Autodesk Inventor part; units mm, degrees
ref_plane "YZ Plane" through (0, 0, 0) normal (1, 0, 0) x (0, 1, 0)
ref_plane "XZ Plane" through (0, 0, 0) normal (0, 1, 0) x (-1, 0, 0)
ref_plane "XY Plane" through (0, 0, 0) normal (0, 0, 1) x (1, 0, 0)
sketch "Sketch1" plane through (0, 0, 0) normal (0, 1, 0) x (-1, 0, 0)
  line L0 (0, 0) -> (0, 20.8)
  line L1 (0, 20.8) -> (-2, 20.8)
  line L2 (-2, 20.8) -> (-2, 14.8)
  line L3 (-2, 14.8) -> (-3, 14.8)
  line L4 (-3, 14.8) -> (-3, 2.8)
  line L5 (-3, 2.8) -> (-5, 2.8)
  line L6 (-5, 2.8) -> (-5, 0)
  line L7 (-5, 0) -> (0, 0)
  dimension "d0" = 10
  dimension "d1" = 6
  dimension "d2" = 4
  dimension "d3" = 6
  dimension "d4" = 12
  dimension "d5" = 2.8
revolve "Revolution1" add sketch "Sketch1" angle 360 about axis through (0, 0, 0) along (0, 0, 1)
thread "Thread1"
sketch "Sketch2" plane through (0, 0, 0) normal (0, 0, -1) x (-1, 0, 0)
  line L0 (0, 1.4434) -> (1.25, 0.7217)
  line L1 (1.25, 0.7217) -> (1.25, -0.7217)
  line L2 (1.25, -0.7217) -> (0, -1.4434)
  line L3 (0, -1.4434) -> (-1.25, -0.7217)
  line L4 (-1.25, -0.7217) -> (-1.25, 0.7217)
  line L5 (-1.25, 0.7217) -> (0, 1.4434)
  point P0 (0, 0)
  point P1 (0, 0)
  dimension "d9" = 2.5
extrude "Extrusion1" cut sketch "Sketch2" against normal blind 2
chamfer "Chamfer1" distance 0.43 angle 45 1 edges at (-2, 0, 20.8)
properties part number "DBTSY4-12-6-DHC" material "Stainless Steel AISI 304"
Model file for the job. Use its own axes, mm. A direction names the side the tool comes from. Give positions to 0.01 mm unless a question says otherwise; leave off trailing zeros. Order: outer loops, then holes, each group sorted by start corner. A loop starts at its lowest first (then second) coordinate and runs counter-clockwise, first axis right, second up. Notation, with made-up numbers: (20.5, 45.25) - (34.5, 45.25) arc R24 cw to (34.5, 80.25) - close; hole circle Ø10 at (-12.75, 27). An arc over 180 degrees is marked (long way). Return JSON: item names as keys, results as strings.
1) Cut at D-D, the plane y = 4. Give the cut face in (x, z).
Geometry says:
{"outline": "(-3, 0) - (3, 0) - (3, 2.8) - (-3, 2.8) - close"}
2) Pull direction X, two halves, no side cores. Call faces 4 (the cylindrical face through (-3, 0, 9)), 5 (the flat face through (-0.616, 1.088, 0.986)), 6 (the flat face through (1, -2, 14.8)): pulls with the +X half, pulls with the -X half, needs draft (parallel to the pull), parting line crosses it, or undercut.
Geometry says:
{"face 4": "parting line crosses it", "face 5": "undercut", "face 6": "needs draft"}
3) 3-axis set-ups, long thin cutter, end or side, ignore diameter. For faces 1 (the flat face through (0, 0, 2)), 2 (the flat face through (0, 0, 20.8)), 3 (the cylindrical face through (0, 2, 18)): which of +Z, -Z, +X, -X, +Y, -Y reach the whole face in a straight line?
Geometry says:
{"face 1": "-Z", "face 2": "+Z, +X, -X, +Y, -Y", "face 3": "+Z"}
4) Cut at C-C, the plane x = -3.25. Give the cut face in (y, z).
Geometry says:
{"outline": "(-3.8, 0) - (3.8, 0) - (3.8, 2.8) - (-3.8, 2.8) - close"}
5) Cut at A-A, the plane y = 0. Give the cut face in (x, z), plus the area to 3 significant figures.
Geometry says:
{"outline": "(-5, 0) - (-1.25, 0) - (-1.25, 2) - (1.25, 2) - (1.25, 0) - (5, 0) - (5, 2.8) - (3, 2.8) - (3, 14.8) - (2, 14.8) - (2, 20.37) - (1.57, 20.8) - (-1.57, 20.8) - (-2, 20.37) - (-2, 14.8) - (-3, 14.8) - (-3, 2.8) - (-5, 2.8) - close", "area": "119 mm²"}
6) Flat gauge pin, fed straight in: P1, Ø0.8, axis at x = 0, y = 0.5, coming from the -Z side. Where does the tip first touch, or does it go through?
Geometry says:
{"P1": "z = 2"}
7) Cut at B-B, the plane z = 17.75. Give the cut face in (x, y).
Geometry says:
{"outline": "circle Ø4 at (0, 0)"}
8) Probe line 1 (Y direction, x = 0, z = 12.5); line 2 (Z direction, x = -1, y = 4.5); line 3 (X direction, y = 0.5, z = 17). List the from-to ranges inside material, lowest first. Write a range as from..to.
Geometry says:
{"line 1": "-3..3", "line 2": "0..2.8", "line 3": "-1.94..1.94"}
